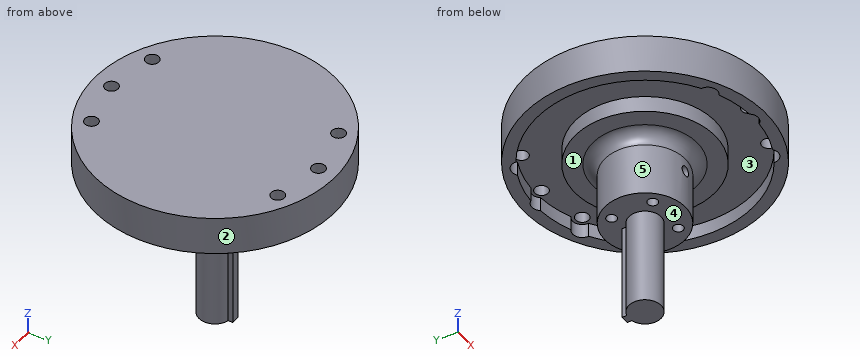
from build123d import *

# Parameters (mm, degrees)
SKETCH1_W                  = 30
SKETCH1_H                  = 9.5
CUT_EXTRUDE1_DEPTH         = 3.5
SKETCH3_R                  = 17.4
BOSS_EXTRUDE1_DEPTH        = 4
SKETCH4_R                  = 10
BOSS_EXTRUDE2_DEPTH        = 16
CUT_EXTRUDE2_DEPTH         = 50.759421218
SKETCH6_W                  = 4
SKETCH6_H                  = 26
F_4_CLEARANCE_HOLE1_D      = 3.3
F_2_CLEARANCE_HOLE1_D      = 2.5
F_2_CLEARANCE_HOLE1_DEPTH  = 12
F_2_CLEARANCE_HOLE2_REACH  = 54.582
F_2_CLEARANCE_HOLE2_BORE_R = 1.25
F_2_CLEARANCE_HOLE3_D      = 2.5
F_2_CLEARANCE_HOLE3_DEPTH  = 40
FILLET1_R                  = 3
EXTRUDE_1_DEPTH            = 50


with BuildPart() as part:
    # Sketch1 → Revolve1 (revolve)
    with BuildSketch(Plane.XZ, mode=Mode.PRIVATE) as revolve1_sk:
        with Locations((15, 5.25)):
            Rectangle(SKETCH1_W, SKETCH1_H)
    revolve(revolve1_sk.sketch.rotate(Axis((0, 0, 10), (0, 0, -1)), 180), axis=Axis((0, 0, 10), (0, 0, -1)))

    # Sketch2 → Cut-Extrude1 (cut)
    with BuildSketch(Plane(origin=(0, 0, 0.5), x_dir=(-1, 0, 0), z_dir=(0, 0, -1))):
        with BuildLine():
            ThreePointArc((1.901854596, -26.932934283), (6.318658968, -26.250229501), (10.562335147, -24.848281153))
            ThreePointArc((10.562335147, -24.848281153), (13.103370267, -25.060195635), (14.379253383, -22.852506912))
            ThreePointArc((14.379253383, -22.852506912), (27, 0), (14.379253383, 22.852506912))
            ThreePointArc((14.379253383, 22.852506912), (13.103370267, 25.060195635), (10.562335147, 24.848281153))
            ThreePointArc((10.562335147, 24.848281153), (6.318658968, 26.250229501), (1.901854596, 26.932934283))
            ThreePointArc((1.901854596, 26.932934283), (0, 27.88125), (-1.901854596, 26.932934283))
            ThreePointArc((-1.901854596, 26.932934283), (-6.318658968, 26.250229501), (-10.562335147, 24.848281153))
            ThreePointArc((-10.562335147, 24.848281153), (-13.103370267, 25.060195635), (-14.379253383, 22.852506912))
            ThreePointArc((-14.379253383, 22.852506912), (-27, 0), (-14.379253383, -22.852506912))
            ThreePointArc((-14.379253383, -22.852506912), (-13.103370267, -25.060195635), (-10.562335147, -24.848281153))
            ThreePointArc((-10.562335147, -24.848281153), (-6.318658968, -26.250229501), (-1.901854596, -26.932934283))
            ThreePointArc((-1.901854596, -26.932934283), (0, -27.88125), (1.901854596, -26.932934283))
        make_face()
    extrude(amount=-CUT_EXTRUDE1_DEPTH, mode=Mode.SUBTRACT)

    # Sketch3 → Boss-Extrude1 (add)
    with BuildSketch(Plane(origin=(0, 0, 4), x_dir=(-1, 0, 0), z_dir=(0, 0, -1))):
        Circle(SKETCH3_R)
    extrude(amount=BOSS_EXTRUDE1_DEPTH)

    # Sketch4 → Boss-Extrude2 (add)
    with BuildSketch(Plane(origin=(0, 0, 0), x_dir=(-1, 0, 0), z_dir=(0, 0, -1))):
        Circle(SKETCH4_R)
    extrude(amount=BOSS_EXTRUDE2_DEPTH)

    # Sketch5 → Cut-Extrude2 (cut, through all)
    with BuildSketch(Plane.XY.offset(10)):
        with BuildLine():
            Line((1, 5), (-1, 5))
            Line((-1, 5), (-1, 3.872983346))
            ThreePointArc((-1, 3.872983346), (0, 4), (1, 3.872983346))
            Line((1, 3.872983346), (1, 5))
        make_face()
    extrude(amount=-CUT_EXTRUDE2_DEPTH, mode=Mode.SUBTRACT)

    # Sketch6 → Cut-Revolve1 (revolve, cut)
    with BuildSketch(Plane.XZ):
        with Locations((2, -3)):
            Rectangle(SKETCH6_W, SKETCH6_H)
    revolve(axis=Axis((0, 0, 10), (0, 0, -1)), mode=Mode.SUBTRACT)

    # #4 Clearance Hole1 (through all)
    with Locations(Plane(origin=(0, 0, 4), x_dir=(-1, 0, 0), z_dir=(0, 0, -1))):
        with Locations((12, -22.95), (0, -25.5), (-12, -22.95), (-12, 22.95), (0, 25.5), (12, 22.95)):
            Hole(F_4_CLEARANCE_HOLE1_D / 2)

    # #2 Clearance Hole1
    with Locations(Plane(origin=(0, 0, -16), x_dir=(-1, 0, 0), z_dir=(0, 0, -1))):
        with Locations((-5.055813485, -5.055813485), (5.055813485, -5.055813485), (5.055813485, 5.055813485), (-5.055813485, 5.055813485)):
            Hole(F_2_CLEARANCE_HOLE1_D / 2, depth=F_2_CLEARANCE_HOLE1_DEPTH)

    # #2 Clearance Hole2 bore (on position points) → #2 Clearance Hole2 (cut, up to next)
    with BuildSketch(Plane(origin=(0, -10, -6.276306458), x_dir=(-1, 0, 0), z_dir=(0, -1, 0)), mode=Mode.PRIVATE) as f_2_clearance_hole2_sk1:
        Circle(F_2_CLEARANCE_HOLE2_BORE_R)
    f_2_clearance_hole2_tool1 = extrude(f_2_clearance_hole2_sk1.sketch, amount=-F_2_CLEARANCE_HOLE2_REACH, mode=Mode.PRIVATE) & part.part
    add(f_2_clearance_hole2_tool1.solids().sort_by_distance((0, -10, -6.276306))[0], mode=Mode.SUBTRACT)

    # #2 Clearance Hole3
    with Locations(Plane(origin=(0, 10, -6.276306458), x_dir=(1, 0, 0), z_dir=(0, 1, 0))):
        with Locations((0, 0)):
            Hole(F_2_CLEARANCE_HOLE3_D / 2, depth=F_2_CLEARANCE_HOLE3_DEPTH)

    # Fillet1
    fillet1_edges = [part.edges().sort_by_distance(p)[0] for p in [
        (10, 0, 0),
    ]]
    fillet(fillet1_edges, radius=FILLET1_R)

    # 草图1 → 凸台-拉伸1 (add)
    with BuildSketch(Plane.XY.offset(10)):
        with BuildLine():
            Line((-1, 5), (-1, 3.872983346))
            ThreePointArc((-1, 3.872983346), (0, -4), (1, 3.872983346))
            Line((1, 3.872983346), (1, 5))
            Line((1, 5), (-1, 5))
        make_face()
    extrude(amount=-EXTRUDE_1_DEPTH)


solid = part.part
Design review of the part built by this model. Coordinates are the model's own, in mm. Face numbers are marked on the shaded views. A direction names the side the tool comes from. Round coordinates to 2 decimals unless told otherwise and drop trailing zeros. Write each loop counter-clockwise with the first axis right and the second up, starting at its lowest first coordinate (ties: lowest second). Pieces come first, ordered by that corner, then holes. Notation, with made-up numbers: (14, 2) - (70, 2) arc R12 cw to (70, 15) - close; hole circle Ø7 at (59, -36). An arc over 180 degrees is marked (long way). Use a Markdown table: item, result. Add a question column.
1. Clearance check with flat-ended pins moving along their axes: pin 1 (4 mm diameter, centred on x = 5.06, y = 5.06, fed in from -Z); pin 2 (3 mm diameter, centred on x = 0, z = -6.28, fed in from -Y); pin 3 (6 mm diameter, centred on y = -6, z = -10, fed in from +X); pin 4 (10 mm diameter, centred on x = -5, y = 4, fed in from -Z). State where each tip first meets the part, or that it passes through.
2. We need section D-D (x = 20). State the section outline as (y, z) points, then the cut area to 3 significant figures.
3. For the marked faces 1 and 2, list the 3-axis set-ups (+Z, -Z, +X, -X, +Y, -Y) from which the entire face can be reached by the end or side of a thin tool; tool diameter is ignored.
4. We need section B-B (x = 0). Count the separate pieces of the cut face and the enclosed holes in it, then the cut area to 3 significant figures.
5. Wall thickness on probe 1 along X at (y, z) = (6, -8); probe 2 along X at (y, z) = (-22, 6); probe 3 along Y at (x, z) = (12, 6.7): over which ranges is each line inside the solid? List them lowest first.
6. We need section A-A (y = 0). State the section outline as (x, z) points.
7. We need section C-C (z = -30.5). State the section outline as (x, y) points.
8. Mouldability with a two-part tool opening along Y and no side actions: class the marked faces 3, 4 and 5 as +Y half, -Y half, draft (parallel to the pull), parting line (faces both ways), or undercut.
Output:
| question | item | result |
|---|---|---|
| 1 | pin 1 | stops at z = -16 |
| 1 | pin 2 | stops at y = -10 |
| 1 | pin 3 | stops at x = 9.54 |
| 1 | pin 4 | stops at z = -40 |
| 2 | outline | (-22.36, 0.5) - (-18.14, 0.5) - (-18.14, 4) - (18.14, 4) - (18.14, 0.5) - (22.36, 0.5) - (22.36, 10) - (-22.36, 10) - close |
| 2 | area | 298 mm2 |
| 3 | face 1 | -Z |
| 3 | face 2 | +Z, -Z |
| 4 | separate pieces | 3 |
| 4 | enclosed holes | 0 |
| 4 | area | 987 mm2 |
| 5 | probe 1 | x = -8 to -5.87, -4.24 to 4.24, 5.87 to 8 |
| 5 | probe 2 | x = -20.4 to -13.35, -10.65 to 10.65, 13.35 to 20.4 |
| 5 | probe 3 | y = -27.5 to -24.6, -21.3 to 21.3, 24.6 to 27.5 |
| 6 | outline | (-30, 0.5) - (-27, 0.5) - (-27, 4) - (-17.4, 4) - (-17.4, 0) - (-13, 0) arc R3 cw to (-10, -3) - (-10, -16) - (-4, -16) - (-4, -40) - (4, -40) - (4, -16) - (10, -16) - (10, -3) arc R3 cw to (13, 0) - (17.4, 0) - (17.4, 4) - (27, 4) - (27, 0.5) - (30, 0.5) - (30, 10) - (-30, 10) - close |
| 7 | outline | (-1, 3.87) arc R4 ccw (long way) to (1, 3.87) - (1, 5) - (-1, 5) - close |
| 8 | face 3 | undercut |
| 8 | face 4 | draft |
| 8 | face 5 | parting line |
